Source: CAD feature listing. Evaluate the final solid. Frame: model axes, mm. Round coordinates to 2 decimals unless told otherwise and drop trailing zeros. Loops run counter-clockwise (first coordinate to the right, second up) from the corner with the lowest first, then second, coordinate; pieces in that order, holes last. Notation, with made-up numbers: M 55,15.5 L 75,15.5 A6 cw 75,24.5 Z; hole C 53.25,66.25 d11. An arc over 180 degrees is marked long. Answer as a JSON object with one key per item and string values.
from build123d import *

# Parameters (mm, degrees)
SKETCH_1_R      = 6
SKETCH_1_R_2    = 2.75
EXTRUDE_1_DEPTH = 18


with BuildPart() as part:
    # 草图1 → 凸台-拉伸1 (new body)
    with BuildSketch(Plane.XY):
        with BuildLine():
            Line((-17.5, 0), (-17.5, -40))
            Line((-17.5, -40), (17.5, -40))
            Line((17.5, -40), (17.5, 0))
            ThreePointArc((17.5, 0), (0, 17.5), (-17.5, 0))
        make_face()
        Circle(SKETCH_1_R, mode=Mode.SUBTRACT)
        with Locations((-10, -30)):
            Circle(SKETCH_1_R_2, mode=Mode.SUBTRACT)
        with Locations((10, -30)):
            Circle(SKETCH_1_R_2, mode=Mode.SUBTRACT)
    extrude(amount=EXTRUDE_1_DEPTH)


solid = part.part
Item 1: Section D-D on y = -3.5. Return the cut outline in (x, z).
Answer sheet:
{"outline": "M -17.5,0 L -4.87,0 L -4.87,18 L -17.5,18 Z; M 4.87,0 L 17.5,0 L 17.5,18 L 4.87,18 Z"}
Item 2: Section B-B on z = 15.5. Return the cut outline in (x, y), then the cut area to 3 significant figures.
Answer sheet:
{"outline": "M -17.5,-40 L 17.5,-40 L 17.5,0 A17.5 ccw -17.5,0 Z; hole C -10,-30 d5.5; hole C 0,0 d12; hole C 10,-30 d5.5", "area": "1,720 mm²"}
Item 3: Section C-C on x = -8. Return the cut outline in (y, z).
Answer sheet:
{"outline": "M -40,0 L -31.89,0 L -31.89,18 L -40,18 Z; M -28.11,0 L 15.56,0 L 15.56,18 L -28.11,18 Z"}
Item 4: Line query: probe 1 along Y at (x, z) = (0, 10.75); probe 2 along X at (y, z) = (-28, 17); probe 3 along Y at (x, z) = (11.5, 2.75). Output: solid intervals per line, ascending. Write a range as from..to.
Answer sheet:
{"probe 1": "y = -40..-6, 6..17.5", "probe 2": "x = -17.5..-11.89, -8.11..8.11, 11.89..17.5", "probe 3": "y = -40..-32.3, -27.7..13.19"}
Item 5: Pull-direction query (Y, two-part tool) for faces 1 (the flat face through (17.5, -20, 9)), 2 (the cylindrical face through (9.642, -27.273, 8.874)), 3 (the cylindrical face through (0.385, 17.496, 8.874)), 4 (the flat face through (0, -40, 9)); classes: pulls with the +Y half, pulls with the -Y half, needs draft (parallel to the pull), parting line crosses it, or undercut.
Answer sheet:
{"face 1": "needs draft", "face 2": "undercut", "face 3": "pulls with the +Y half", "face 4": "pulls with the -Y half"}
Item 6: Section A-A on y = -30. Return the cut outline in (x, z), then the cut area to 3 significant figures.
Answer sheet:
{"outline": "M -17.5,0 L -12.75,0 L -12.75,18 L -17.5,18 Z; M -7.25,0 L 7.25,0 L 7.25,18 L -7.25,18 Z; M 12.75,0 L 17.5,0 L 17.5,18 L 12.75,18 Z", "area": "432 mm²"}
Item 7: Contact query for flat-ended pins moving along their axis: pin 1 Ø10 at (x, z) = (-9.5, 3.5) entering from +Y; pin 2 Ø4 at (y, z) = (11.5, 6.5) entering from +X. Output: stop coordinate, or through.
Answer sheet:
{"pin 1": "stops at y = 16.91", "pin 2": "stops at x = 14.7"}
